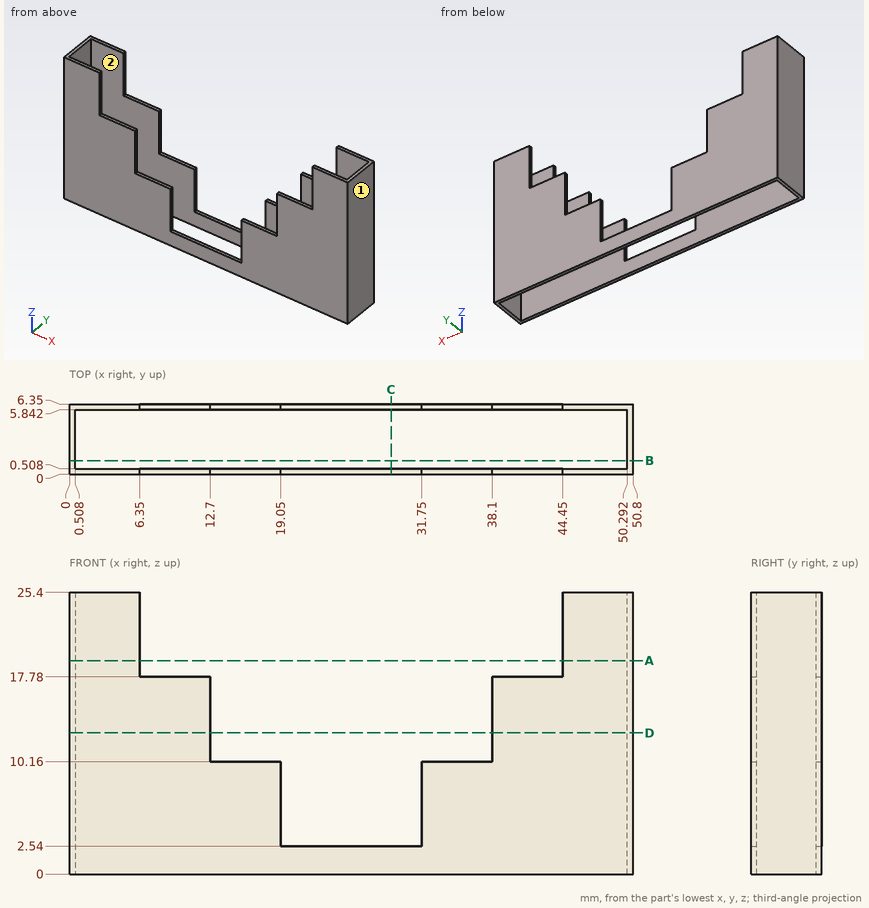
Verification items for this drawing (mm, ordinates from the low corner). A direction names the side the tool comes from. Give positions to 0.01 mm unless a question says otherwise; leave off trailing zeros. Write each loop counter-clockwise with the first axis right and the second up, starting at its lowest first coordinate (ties: lowest second). Pieces come first, ordered by that corner, then holes.
1) Section check B-B, the plane y = 1.25. Record the boundary of the cut face in (x, z), and give its area (3 significant figures).
2) Section check C-C, the plane x = 29. Record the boundary of the cut face in (y, z).
3) Gauge pin test, flat ends, axial feed: pin 1 (0.6 mm diameter, centred on x = 23, y = 6, fed in from +Z); pin 2 (0.6 mm diameter, centred on x = 41.5, y = 6, fed in from +Z). Record the tip position at first contact, or that the pin passes through.
4) Material ranges on L1, parallel to Y at x = 5, z = 17; L2, parallel to X at y = 1.75, z = 12.75; L3, parallel to Z at x = 27.5, y = 6, recorded low to high.
5) Access from +Z, -Z, +X, -X, +Y, -Y to the whole of each face (thin tool, end or side, straight path). Record for the marked faces 1 and 2.
6) Section check A-A, the plane z = 19.25. Record the boundary of the cut face in (x, y), and give its area (3 significant figures).
7) Section check D-D, the plane z = 12.75. Record the boundary of the cut face in (x, y), and give its area (3 significant figures).
Computed:
1. outline: (0, 0) - (0.51, 0) - (0.51, 25.4) - (0, 25.4) - close; (50.29, 0) - (50.8, 0) - (50.8, 25.4) - (50.29, 25.4) - close
1. area: 25.8 mm2
2. outline: (0, 0) - (0.51, 0) - (0.51, 2.54) - (0, 2.54) - close; (5.84, 0) - (6.35, 0) - (6.35, 2.54) - (5.84, 2.54) - close
3. pin 1: stops at z = 2.54
3. pin 2: stops at z = 17.78
4. L1: y = 0 to 0.51, 5.84 to 6.35
4. L2: x = 0 to 0.51, 50.29 to 50.8
4. L3: z = 0 to 2.54
5. face 1: +Z, -Z, +X, +Y, -Y
5. face 2: +Z, -Z
6. outline: (0, 0) - (6.35, 0) - (6.35, 0.51) - (0.51, 0.51) - (0.51, 5.84) - (6.35, 5.84) - (6.35, 6.35) - (0, 6.35) - close; (44.45, 0) - (50.8, 0) - (50.8, 6.35) - (44.45, 6.35) - (44.45, 5.84) - (50.29, 5.84) - (50.29, 0.51) - (44.45, 0.51) - close
6. area: 18.3 mm2
7. outline: (0, 0) - (12.7, 0) - (12.7, 0.51) - (0.51, 0.51) - (0.51, 5.84) - (12.7, 5.84) - (12.7, 6.35) - (0, 6.35) - close; (38.1, 0) - (50.8, 0) - (50.8, 6.35) - (38.1, 6.35) - (38.1, 5.84) - (50.29, 5.84) - (50.29, 0.51) - (38.1, 0.51) - close
7. area: 31.2 mm2
